Geometry check sheet. Reference: the model listing, model coordinates, mm. Round coordinates to 2 decimals unless told otherwise and drop trailing zeros. Write each loop counter-clockwise with the first axis right and the second up, starting at its lowest first coordinate (ties: lowest second). Pieces come first, ordered by that corner, then holes. Notation, with made-up numbers: M -37,-18 L 8,-18 A22 ccw 8,-2 Z; hole C -5.5,37 d8. An arc over 180 degrees is marked long. Answer in a Markdown table with one row per item. Add a question column.
from build123d import *

# Parameters (mm, degrees)
F0_W     = 100
F0_H     = 160
F1_DEPTH = 6.45
F3_D     = 8.8
F5_D     = 4.9784
F7_D     = 28.575


with BuildPart() as f1:
    # F0 (on Top) → F1 (new body)
    with BuildSketch(Plane.XY):
        Rectangle(F0_W, F0_H)
    extrude(amount=F1_DEPTH)

    # F3 (through all)
    with Locations(Plane.XY.offset(6.45)):
        with Locations((-22.5, 57.5), (22.5, 57.5), (22.5, 12.5), (-22.5, 12.5)):
            Hole(F3_D / 2)

    # F5 (through all)
    with Locations(Plane.XY.offset(6.45)):
        with Locations((-15.4149278299, -32.0850721701), (15.4149278299, -32.0850721701), (15.4149278299, -62.9149278299), (-15.4149278299, -62.9149278299)):
            Hole(F5_D / 2)

    # F7 (through all)
    with Locations(Plane.XY.offset(6.45)):
        with Locations((0, -47.5)):
            Hole(F7_D / 2)


solid = f1.part
Item 1: Mould release check, pull along Y, two halves, no side actions. Record for faces 1 (the flat face through (-1, -80, 3)), 2 (the flat face through (50, -1, 3)), 3 (the cylindrical face through (-21.546, 53.205, 3.18)): +Y half, -Y half, draft (parallel to the pull), parting line (faces both ways), or undercut.
Item 2: Section check D-D, the plane x = 0. Record the boundary of the cut face in (y, z), and give its area (3 significant figures).
Item 3: Section check B-B, the plane x = 22.5. Record the boundary of the cut face in (y, z), and give its area (3 significant figures).
Item 4: Gauge pin test, flat ends, axial feed: pin 1 Ø10 at (x, y) = (22.5, 12.5) entering from -Z; pin 2 Ø7 at (x, y) = (-22.5, 12.5) entering from +Z. Record the tip position at first contact, or that the pin passes through.
Item 5: Scan lines: probe 1 along Y at (x, z) = (22.5, 2); probe 2 along Y at (x, z) = (15.5, 0.75); probe 3 along X at (y, z) = (10, 1). Record each from-to range of solid material in increasing order. Write a range as from..to.
Item 6: Section check C-C, the plane y = -47.5. Record the boundary of the cut face in (x, z).
Item 7: Section check A-A, the plane y = 57.5. Record the boundary of the cut face in (x, z).
Result sheet:
| question | item | result |
|---|---|---|
| 1 | face 1 | -Y half |
| 1 | face 2 | draft |
| 1 | face 3 | undercut |
| 2 | outline | M -80,0 L -61.79,0 L -61.79,6.45 L -80,6.45 Z; M -33.21,0 L 80,0 L 80,6.45 L -33.21,6.45 Z |
| 2 | area | 848 mm^2 |
| 3 | outline | M -80,0 L 8.1,0 L 8.1,6.45 L -80,6.45 Z; M 16.9,0 L 53.1,0 L 53.1,6.45 L 16.9,6.45 Z; M 61.9,0 L 80,0 L 80,6.45 L 61.9,6.45 Z |
| 3 | area | 918 mm^2 |
| 4 | pin 1 | stops at z = 0 |
| 4 | pin 2 | passes through |
| 5 | probe 1 | y = -80..8.1, 16.9..53.1, 61.9..80 |
| 5 | probe 2 | y = -80..-65.4, -60.43..-34.57, -29.6..80 |
| 5 | probe 3 | x = -50..-26.12, -18.88..18.88, 26.12..50 |
| 6 | outline | M -50,0 L -14.29,0 L -14.29,6.45 L -50,6.45 Z; M 14.29,0 L 50,0 L 50,6.45 L 14.29,6.45 Z |
| 7 | outline | M -50,0 L -26.9,0 L -26.9,6.45 L -50,6.45 Z; M -18.1,0 L 18.1,0 L 18.1,6.45 L -18.1,6.45 Z; M 26.9,0 L 50,0 L 50,6.45 L 26.9,6.45 Z |
